from build123d import *

# Parameters (mm, degrees)
EXTRUDE_1_DEPTH             = 10
M4X0_71_D                   = 3.3
M4X0_71_DEPTH               = 19
M4X0_71_TIP                 = 0.991420021
M4X0_72_D                   = 3.3
M4X0_72_DEPTH               = 19
M4X0_72_TIP                 = 0.991420021
FILLET_1_R                  = 2
FILLET_2_R                  = 4
CHAMFER_1_SIZE              = 1
HOLE_WIZARD_M41_D           = 4.5
HOLE_WIZARD_M41_CBORE_D     = 8
HOLE_WIZARD_M41_CBORE_DEPTH = 4


with BuildPart() as part:
    # Эскиз1 → Бобышка-Вытянуть1 (new body)
    with BuildSketch(Plane.XY):
        with BuildLine():
            Line((-44.995331881, 7.495331881), (-57.250992251, -4.76032849))
            Line((-57.250992251, -4.76032849), (-51.169873933, -10.841446808))
            Line((-51.169873933, -10.841446808), (-44.098806121, -3.770378996))
            ThreePointArc((-44.098806121, -3.770378996), (-32.125988463, 5.374011537), (-41.270378996, -6.598806121))
            Line((-41.270378996, -6.598806121), (-48.341446808, -13.669873933))
            Line((-48.341446808, -13.669873933), (-42.26032849, -19.750992251))
            Line((-42.26032849, -19.750992251), (-30.004668119, -7.495331881))
            ThreePointArc((-30.004668119, -7.495331881), (-27.706876955, -4.056444383), (-26.9, 0))
            Line((-26.9, 0), (-22.3, 4.6))
            Line((-22.3, 4.6), (22.3, 4.6))
            Line((22.3, 4.6), (26.9, 0))
            ThreePointArc((26.9, 0), (27.706876955, -4.056444383), (30.004668119, -7.495331881))
            Line((30.004668119, -7.495331881), (42.26032849, -19.750992251))
            Line((42.26032849, -19.750992251), (48.341446808, -13.669873933))
            Line((48.341446808, -13.669873933), (41.270378996, -6.598806121))
            ThreePointArc((41.270378996, -6.598806121), (32.125988463, 5.374011537), (44.098806121, -3.770378996))
            Line((44.098806121, -3.770378996), (51.169873933, -10.841446808))
            Line((51.169873933, -10.841446808), (57.250992251, -4.76032849))
            Line((57.250992251, -4.76032849), (44.995331881, 7.495331881))
            ThreePointArc((44.995331881, 7.495331881), (41.556444383, 9.793123045), (37.5, 10.6))
            Line((37.5, 10.6), (-37.5, 10.6))
            ThreePointArc((-37.5, 10.6), (-41.556444383, 9.793123045), (-44.995331881, 7.495331881))
        make_face()
    extrude(amount=EXTRUDE_1_DEPTH)

    # Отверстие обработанное метчиком M4x0.71
    with Locations(Plane(origin=(11.254668119, 11.254668119, 0), x_dir=(0, 0, 1), z_dir=(-0.707106781, -0.707106781, 0))):
        with Locations((5, -38.848625406)):
            Hole(M4X0_71_D / 2, depth=M4X0_71_DEPTH)
            with Locations((0, 0, -(M4X0_71_DEPTH + M4X0_71_TIP / 2))):  # 118° drill point
                Cone(0, M4X0_71_D / 2, M4X0_71_TIP, mode=Mode.SUBTRACT)

    # Отверстие обработанное метчиком M4x0.72
    with Locations(Plane(origin=(-11.254668119, 11.254668119, 0), x_dir=(0, 0, -1), z_dir=(0.707106781, -0.707106781, 0))):
        with Locations((-5, -38.848625406)):
            Hole(M4X0_72_D / 2, depth=M4X0_72_DEPTH)
            with Locations((0, 0, -(M4X0_72_DEPTH + M4X0_72_TIP / 2))):  # 118° drill point
                Cone(0, M4X0_72_D / 2, M4X0_72_TIP, mode=Mode.SUBTRACT)

    # Скругление1
    fillet_1_edges = [part.edges().sort_by_distance(p)[0] for p in [
        (-42.26032849, -19.750992251, 5),
        (-48.341446808, -13.669873933, 5),
        (-41.270378996, -6.598806121, 5),
        (-44.098806121, -3.770378996, 5),
        (-51.169873933, -10.841446808, 5),
        (-57.250992251, -4.76032849, 5),
        (57.250992251, -4.76032849, 5),
        (51.169873933, -10.841446808, 5),
        (44.098806121, -3.770378996, 5),
        (41.270378996, -6.598806121, 5),
        (48.341446808, -13.669873933, 5),
        (42.26032849, -19.750992251, 5),
    ]]
    fillet(fillet_1_edges, radius=FILLET_1_R)

    # Скругление2
    fillet_2_edges = [part.edges().sort_by_distance(p)[0] for p in [
        (26.9, 0, 5),
        (22.3, 4.6, 5),
        (-22.3, 4.6, 5),
        (-26.9, 0, 5),
    ]]
    fillet(fillet_2_edges, radius=FILLET_2_R)

    # Фаска1
    chamfer_1_edges = [part.edges().sort_by_distance(p)[0] for p in [
        (-41.268947779, -7.045325886, 10),
        (-44.545325886, -3.768947779, 10),
        (41.268947779, -7.045325886, 10),
        (44.545325886, -3.768947779, 10),
        (47.513019683, -13.669873933, 10),
        (42.26032849, -18.922565126, 10),
        (51.169873933, -10.013019683, 10),
        (56.422565126, -4.76032849, 10),
        (-24.653465253, 2.246534747, 0),
        (-24.653465253, 2.246534747, 10),
        (0, 4.6, 0),
        (0, 4.6, 10),
        (27.970298296, -4.641636073, 0),
        (27.970298296, -4.641636073, 10),
        (24.653465253, 2.246534747, 0),
        (24.653465253, 2.246534747, 10),
        (-26.603044357, -0.012223974, 0),
        (-26.603044357, -0.012223974, 10),
        (-22.17387948, 4.29551813, 0),
        (-22.17387948, 4.29551813, 10),
        (26.603044357, -0.012223974, 0),
        (26.603044357, -0.012223974, 10),
        (22.17387948, 4.29551813, 0),
        (22.17387948, 4.29551813, 10),
        (35.425391524, -12.916055285, 10),
        (-50.416055285, 2.074608476, 0),
        (-41.556444383, 9.793123045, 0),
        (0, 10.6, 0),
        (41.556444383, 9.793123045, 0),
        (35.425391524, -12.916055285, 0),
        (-27.970298296, -4.641636073, 0),
        (-27.970298296, -4.641636073, 10),
        (41.556444383, 9.793123045, 10),
        (0, 10.6, 10),
        (-41.556444383, 9.793123045, 10),
        (-50.416055285, 2.074608476, 10),
        (50.416055285, 2.074608476, 0),
        (50.416055285, 2.074608476, 10),
        (-35.425391524, -12.916055285, 0),
        (-45.300887649, -16.710433092, 0),
        (-44.591959566, -9.920386691, 0),
        (-32.125988463, 5.374011537, 0),
        (-47.420386691, -7.091959566, 0),
        (-54.210433092, -7.800887649, 0),
        (54.210433092, -7.800887649, 0),
        (47.420386691, -7.091959566, 0),
        (32.125988463, 5.374011537, 0),
        (44.591959566, -9.920386691, 0),
        (45.300887649, -16.710433092, 0),
        (-42.26032849, -18.922565126, 0),
        (-47.513019683, -13.669873933, 0),
        (-51.169873933, -10.013019683, 0),
        (-56.422565126, -4.76032849, 0),
        (-41.268947779, -7.045325886, 0),
        (-44.545325886, -3.768947779, 0),
        (41.268947779, -7.045325886, 0),
        (44.545325886, -3.768947779, 0),
        (47.513019683, -13.669873933, 0),
        (42.26032849, -18.922565126, 0),
        (51.169873933, -10.013019683, 0),
        (56.422565126, -4.76032849, 0),
        (54.210433092, -7.800887649, 10),
        (45.300887649, -16.710433092, 10),
        (44.591959566, -9.920386691, 10),
        (32.125988463, 5.374011537, 10),
        (47.420386691, -7.091959566, 10),
        (-54.210433092, -7.800887649, 10),
        (-47.420386691, -7.091959566, 10),
        (-32.125988463, 5.374011537, 10),
        (-44.591959566, -9.920386691, 10),
        (-45.300887649, -16.710433092, 10),
        (-35.425391524, -12.916055285, 10),
        (-42.26032849, -18.922565126, 10),
        (-47.513019683, -13.669873933, 10),
        (-51.169873933, -10.013019683, 10),
        (-56.422565126, -4.76032849, 10),
    ]]
    chamfer(chamfer_1_edges, length=CHAMFER_1_SIZE)

    # Цековка для винта с внутренним шестигранником M41 (through all)
    with Locations(Plane(origin=(0, 4.6, 0), x_dir=(-1, 0, 0), z_dir=(0, -1, 0))):
        with Locations((10, -5), (-10, -5)):
            CounterBoreHole(HOLE_WIZARD_M41_D / 2, HOLE_WIZARD_M41_CBORE_D / 2, HOLE_WIZARD_M41_CBORE_DEPTH)


solid = part.part
Here's how the part is built. I have some questions about the finished solid (model axes, mm). A direction names the side the tool comes from. Round coordinates to 2 decimals unless told otherwise and drop trailing zeros. Write each loop counter-clockwise with the first axis right and the second up, starting at its lowest first coordinate (ties: lowest second). Pieces come first, ordered by that corner, then holes.
1. If we mould it in two halves opening along Z, with no side actions, what happens to faces 5 (the cylindrical face through (51.148, -10.013, 5.056)), 6 (the flat face through (44.93, -16.385, 0.507)), 7 (the flat face through (-53.87, -7.42, 9.51)), 8 (the cylindrical face through (-12.248, 9.614, 4.901))? For each: released by +Z, released by -Z, zero draft, split by the parting line, or undercut.
2. I need wall thicknesses on L1, parallel to X at y = -2.75, z = 9.5; L2, parallel to X at y = -13, z = 4.75; L3, parallel to X at y = 7.75, z = 4. Which ranges of each line are inside material? Lowest first, please.
3. Suppose I cut it at B-B (y = 0). State how many separate pieces and enclosed holes the cut face has, and give its area (3 significant figures).
4. Suppose I cut it at A-A (x = 11). List the corners of the cut face in (y, z) for me.
5. For faces 1 (the flat face through (-12, 8.6, 7)), 2 (the flat face through (-24.7, 2.2, 4.9)), 3 (the flat face through (-43.52, -8.85, 4.94)), 4 (the conical face through (22.298, 4.657, 0.618)), which set-ups out of +Z, -Z, +X, -X, +Y, -Y let a thin tool reach every point of the face, with its end or its side?
6. Will these pins go through, and if not, where does the flat tip stop? pin 1 Ø4 at (x, z) = (-16.5, 3.5) entering from -Y; pin 2 Ø2.5 at (x, z) = (11, 4) entering from -Y; pin 3 Ø2 at (y, z) = (-13, 8) entering from +X.
Answer sheet:
1. face 5: zero draft
1. face 6: released by -Z
1. face 7: released by +Z
1. face 8: undercut
2. L1: x = -54.53 to -45.12, -29.88 to -27.78, 27.78 to 29.88, 45.12 to 54.53
2. L2: x = -47.4 to -44.25, -39.63 to -35.51, 35.51 to 39.63, 44.25 to 47.4
2. L3: x = -44.73 to -13.87, -6.13 to 6.13, 13.87 to 44.73
3. separate pieces: 4
3. enclosed holes: 0
3. area: 205 mm2
4. outline: (4.6, 1) - (5.6, 0) - (9.6, 0) - (10.6, 1) - (10.6, 2.98) - (8.6, 2.98) - (8.6, 1.13) - (4.6, 1.13) - close; (4.6, 8.87) - (8.6, 8.87) - (8.6, 7.02) - (10.6, 7.02) - (10.6, 9) - (9.6, 10) - (5.6, 10) - (4.6, 9) - close
5. face 1: -Y
5. face 2: +Z, -Z, -Y
5. face 3: +Z, -Z
5. face 4: -Z, -Y
6. pin 1: stops at y = 4.6
6. pin 2: stops at y = 8.6
6. pin 3: stops at x = 47.51
